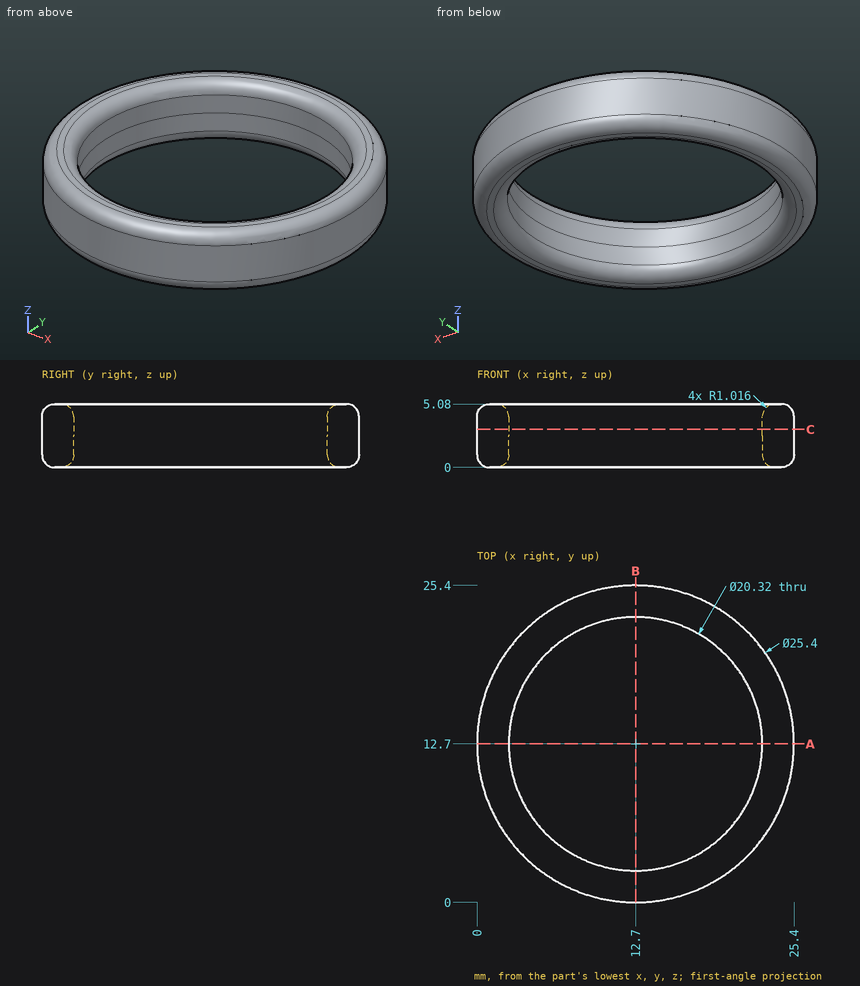
Verification items for this drawing (mm, ordinates from the low corner). Give positions to 0.01 mm unless a question says otherwise; leave off trailing zeros. Loops run counter-clockwise (first coordinate to the right, second up) from the corner with the lowest first, then second, coordinate; pieces in that order, holes last. Notation, with made-up numbers: M 89,18.5 L 116,18.5 A20 ccw 116,22.5 Z; hole C -17.5,42.5 d1. An arc over 180 degrees is marked long. Answer as a JSON object with one key per item and string values. Group by question number.
Item 1: Gauge pin test, flat ends, axial feed: pin 1 (12 mm diameter, centred on x = 12.7, y = 12.7, fed in from -Z); pin 2 (1 mm diameter, centred on x = 19, z = 4.5, fed in from +Y); pin 3 (2 mm diameter, centred on x = 5.5, z = 3.5, fed in from -Y); pin 4 (1 mm diameter, centred on y = 9.5, z = 2.5, fed in from +X). Record the tip position at first contact, or that the pin passes through.
Item 2: Sectioned sample at A-A on y = 12.7. Record the boundary of the cut face in (x, z).
Item 3: Sectioned sample at C-C on z = 3.05. Record the boundary of the cut face in (x, y).
Item 4: Material ranges on L1, parallel to Y at x = 12.7, z = 3.6; L2, parallel to Y at x = 3.75, z = 4; L3, parallel to X at y = 21.25, z = 2.4, recorded low to high.
Findings below:
{
 "1": {"pin 1": "through", "pin 2": "y = 23.95", "pin 3": "y = 1.62", "pin 4": "x = 25.11"},
 "2": {"outline": "M 0,1.02 A1.02 ccw 1.02,0 L 1.52,0 A1.02 ccw 2.54,1.02 L 2.54,4.06 A1.02 ccw 1.52,5.08 L 1.02,5.08 A1.02 ccw 0,4.06 Z; M 22.86,1.02 A1.02 ccw 23.88,0 L 24.38,0 A1.02 ccw 25.4,1.02 L 25.4,4.06 A1.02 ccw 24.38,5.08 L 23.88,5.08 A1.02 ccw 22.86,4.06 Z"},
 "3": {"outline": "C 12.7,12.7 d25.4; hole C 12.7,12.7 d20.32"},
 "4": {"L1": "0 to 2.54, 22.86 to 25.4", "L2": "3.69 to 7.89, 17.51 to 21.71", "L3": "3.31 to 7.21, 18.19 to 22.09"}
}
